Model file for the job. Use its own axes, mm. A direction names the side the tool comes from. Coordinates: 2 decimals unless noted, no trailing zeros. Loops run counter-clockwise (first coordinate to the right, second up) from the corner with the lowest first, then second, coordinate; pieces in that order, holes last. Notation, with made-up numbers: M -32.5,79.25 L -21.5,79.25 A17 ccw -21.5,86.25 Z; hole C 76.5,-35 d6. An arc over 180 degrees is marked long. Write item = value, one per line. Start each with the question number.
from build123d import *

# Parameters (mm, degrees)
SKETCH1_W               = 120
SKETCH1_H               = 50
BODY_DEPTH              = 4
EDGE_FILLETS_R          = 5
GX12_HOLE_D             = 12.5
GX12_NUT_CUT_DEPTH      = 2
GX12_PATTERN_COUNT      = 4
GX12_PATTERN_PITCH      = 24
GX12_PATTERN_COUNT_DIR2 = 2
GX12_PATTERN_PITCH_DIR2 = 24


# Read off the part's stored shape, not the designer's step: mounting_holes
with BuildPart() as part:
    # Sketch1 → body (new body)
    with BuildSketch(Plane(origin=(0, 0, 0), x_dir=(1, 0, 0), z_dir=(0, 1, 0))):
        Rectangle(SKETCH1_W, SKETCH1_H)
    extrude(amount=BODY_DEPTH)

    # mounting_holes outline → mounting_holes (revolve, cut)
    with BuildSketch(Plane(origin=(55, 0, 20), x_dir=(1, 0, 0), z_dir=(0, 0, 1))):
        Polygon((0, 0), (1.7, 0), (1.7, 2), (3.25, 2), (3.25, 3.975), (3.275, 4), (0, 4), align=None)
    revolve(axis=Axis((55, 0, 20), (0, 1, 0)), mode=Mode.SUBTRACT)

    # mounting_holes 2 outline → mounting_holes 2 (revolve, cut)
    with BuildSketch(Plane(origin=(-55, 0, -20), x_dir=(1, 0, 0), z_dir=(0, 0, 1))):
        Polygon((0, 4), (0, 0), (1.7, 0), (1.7, 2), (3.25, 2), (3.25, 3.975), (3.275, 4), align=None)
    revolve(axis=Axis((-55, 0, -20), (0, 1, 0)), mode=Mode.SUBTRACT)

    # mounting_holes 3 outline → mounting_holes 3 (revolve, cut)
    with BuildSketch(Plane(origin=(55, 0, -20), x_dir=(1, 0, 0), z_dir=(0, 0, 1))):
        Polygon((0, 4), (0, 0), (1.7, 0), (1.7, 2), (3.25, 2), (3.25, 3.975), (3.275, 4), align=None)
    revolve(axis=Axis((55, 0, -20), (0, 1, 0)), mode=Mode.SUBTRACT)

    # mounting_holes 4 outline → mounting_holes 4 (revolve, cut)
    with BuildSketch(Plane(origin=(-55, 0, 20), x_dir=(1, 0, 0), z_dir=(0, 0, 1))):
        Polygon((0, 4), (0, 0), (1.7, 0), (1.7, 2), (3.25, 2), (3.25, 3.975), (3.275, 4), align=None)
    revolve(axis=Axis((-55, 0, 20), (0, 1, 0)), mode=Mode.SUBTRACT)

    # edge_fillets
    edge_fillets_edges = [part.edges().sort_by_distance(p)[0] for p in [
        (60, 2, 25),
        (-60, 2, 25),
        (-60, 2, -25),
        (60, 2, -25),
    ]]
    fillet(edge_fillets_edges, radius=EDGE_FILLETS_R)

    # gx12_hole (through all)
    with Locations(Plane(origin=(0, 4, 0), x_dir=(1, 0, 0), z_dir=(0, 1, 0))):
        with Locations((-36, 12)):
            gx12_hole = Hole(GX12_HOLE_D / 2)

    # Sketch6 → gx12_nut_cut (cut)
    with BuildSketch(Plane.XZ):
        Polygon((-36, -3.339745962), (-43.5, -7.669872981), (-43.5, -16.330127019), (-36, -20.660254038), (-28.5, -16.330127019), (-28.5, -7.669872981), align=None)
    gx12_nut_cut = extrude(amount=-GX12_NUT_CUT_DEPTH, mode=Mode.SUBTRACT)

    # gx12_pattern: gx12_hole, gx12_nut_cut 4 × 2
    with Locations(*[(i * GX12_PATTERN_PITCH, 0, j * GX12_PATTERN_PITCH_DIR2) for i in range(GX12_PATTERN_COUNT) for j in range(GX12_PATTERN_COUNT_DIR2) if (i, j) != (0, 0)]):
        add(gx12_hole, mode=Mode.SUBTRACT)
        add(gx12_nut_cut, mode=Mode.SUBTRACT)


solid = part.part
Item 1: Pin check, flat tips, straight feed: pin 1 Ø16.5 at (x, z) = (-33.5, -8.5) entering from -Y; pin 2 Ø3 at (x, z) = (55, -20) entering from +Y; pin 3 Ø7.5 at (x, z) = (12.5, -9.5) entering from -Y; pin 4 Ø5.5 at (x, z) = (55, 20) entering from +Y. Stop position of each tip, or through.
Item 2: Pull direction Z, two halves, no side cores. Call faces 4 (the flat face through (8.303, 0.986, 18.526)), 5 (the flat face through (-28.5, 1, 12)): +Z half, -Z half, draft (parallel to the pull), parting line (faces both ways), or undercut.
Item 3: 3-axis set-ups, long thin cutter, end or side, ignore diameter. For faces 1 (the cylindrical face through (-58.247, 3.001, 19.857)), 2 (the cylindrical face through (53.3, 1.01, 19.93)), 3 (the flat face through (15.697, 0.986, -18.526)): which of +Z, -Z, +X, -X, +Y, -Y reach the whole face in a straight line?
Item 4: Probe L1, parallel to Z at x = -55, y = 3.2; L2, parallel to Z at x = 55, y = 0.6; L3, parallel to X at y = 1.3, z = -14. List the from-to ranges inside material, lowest first.
Item 5: Cut at A-A (x = -31). Give the cut face in (y, z).
Item 6: Cut at B-B (y = 2.95). Give the number of separate pieces and of enclosed holes in the cut face, plus the area to 3 significant figures.
Item 7: Cut at D-D (x = 10). Give the cut face in (y, z).
Reported:
q1.pin_1 = 0
q1.pin_2 = through
q1.pin_3 = 2
q1.pin_4 = 2
q2.face_4 = undercut
q2.face_5 = undercut
q3.face_1 = +Y
q3.face_2 = +Y, -Y
q3.face_3 = -Y
q4.L1 = -25 to -23.25, -16.75 to 16.75, 23.25 to 25
q4.L2 = -25 to -21.7, -18.3 to 18.3, 21.7 to 25
q4.L3 = -60 to -43.5, -28.5 to -19.5, -4.5 to 4.5, 19.5 to 28.5, 43.5 to 60
q5.outline = M 0,-25 L 4,-25 L 4,-15.75 L 2,-15.75 L 2,-17.77 L 0,-17.77 Z; M 0,-6.23 L 2,-6.23 L 2,-8.25 L 4,-8.25 L 4,8.25 L 2,8.25 L 2,6.23 L 0,6.23 Z; M 0,17.77 L 2,17.77 L 2,15.75 L 4,15.75 L 4,25 L 0,25 Z
q6.separate_pieces = 1
q6.enclosed_holes = 12
q6.area = 4,860 mm^2
q7.outline = M 0,-25 L 4,-25 L 4,-17.92 L 2,-17.92 L 2,-19.51 L 0,-19.51 Z; M 0,-4.49 L 2,-4.49 L 2,-6.08 L 4,-6.08 L 4,6.08 L 2,6.08 L 2,4.49 L 0,4.49 Z; M 0,19.51 L 2,19.51 L 2,17.92 L 4,17.92 L 4,25 L 0,25 Z
